```python
from build123d import *

# Parameters (mm, degrees)
SKETCH2_W           = 35.417007692
SKETCH2_H           = 35.417007691
SKETCH2_R           = 1.625
BOSS_EXTRUDE1_DEPTH = 4.975
SKETCH3_R           = 2.5
SKETCH3_R_2         = 1.625
BOSS_EXTRUDE2_DEPTH = 5.4
FILLET1_R           = 2.4
FILLET2_R           = 1


with BuildPart() as part:
    # Sketch2 → Boss-Extrude1 (new body)
    with BuildSketch(Plane.YZ):
        with Locations((28.194, 151.93658674)):
            Rectangle(SKETCH2_W, SKETCH2_H)
        with Locations(Location((16.194, 163.93658674, 0), (0, 0, 270))):
            Circle(SKETCH2_R, mode=Mode.SUBTRACT)
        with Locations(Location((40.194, 163.93658674, 0), (0, 0, 270))):
            Circle(SKETCH2_R, mode=Mode.SUBTRACT)
        with Locations(Location((40.194, 139.93658674, 0), (0, 0, 270))):
            Circle(SKETCH2_R, mode=Mode.SUBTRACT)
        with Locations(Location((16.194, 139.93658674, 0), (0, 0, 270))):
            Circle(SKETCH2_R, mode=Mode.SUBTRACT)
    extrude(amount=BOSS_EXTRUDE1_DEPTH)

    # Sketch3 → Boss-Extrude2 (add)
    # profile 1 of 4: a face of its own
    with BuildSketch(Plane.YZ.offset(4.975)):
        with Locations(Location((16.194, 163.93658674, 0), (0, 0, 90))):
            Circle(SKETCH3_R)
        with Locations(Location((16.194, 163.93658674, 0), (0, 0, 270))):
            Circle(SKETCH3_R_2, mode=Mode.SUBTRACT)
    # profile 2 of 4: a face of its own
    with BuildSketch(Plane.YZ.offset(4.975)):
        with Locations(Location((40.194, 163.93658674, 0), (0, 0, 90))):
            Circle(SKETCH3_R)
        with Locations(Location((40.194, 163.93658674, 0), (0, 0, 270))):
            Circle(SKETCH3_R_2, mode=Mode.SUBTRACT)
    # profile 3 of 4: a face of its own
    with BuildSketch(Plane.YZ.offset(4.975)):
        with Locations(Location((40.194, 139.93658674, 0), (0, 0, 90))):
            Circle(SKETCH3_R)
        with Locations(Location((40.194, 139.93658674, 0), (0, 0, 270))):
            Circle(SKETCH3_R_2, mode=Mode.SUBTRACT)
    # profile 4 of 4: a face of its own
    with BuildSketch(Plane.YZ.offset(4.975)):
        with Locations(Location((16.194, 139.93658674, 0), (0, 0, 90))):
            Circle(SKETCH3_R)
        with Locations(Location((16.194, 139.93658674, 0), (0, 0, 270))):
            Circle(SKETCH3_R_2, mode=Mode.SUBTRACT)
    extrude(amount=BOSS_EXTRUDE2_DEPTH)

    # Fillet1
    fillet1_edges = [part.edges().sort_by_distance(p)[0] for p in [
        (2.4875, 10.485496154, 169.645090586),
        (2.4875, 45.902503846, 169.645090586),
        (2.4875, 45.902503846, 134.228082895),
        (2.4875, 10.485496154, 134.228082895),
    ]]
    fillet(fillet1_edges, radius=FILLET1_R)

    # Fillet2
    fillet2_edges = [part.edges().sort_by_distance(p)[0] for p in [
        (4.975, 16.194, 161.43658674),
        (4.975, 40.194, 161.43658674),
        (4.975, 40.194, 137.43658674),
        (4.975, 16.194, 137.43658674),
        (4.975, 28.194, 169.645090586),
        (4.975, 45.902503846, 151.93658674),
        (4.975, 10.485496154, 151.93658674),
        (4.975, 28.194, 134.228082895),
        (4.975, 11.18843988, 168.942146861),
        (4.975, 11.18843988, 134.93102662),
        (4.975, 45.19956012, 134.93102662),
        (4.975, 45.19956012, 168.942146861),
    ]]
    fillet(fillet2_edges, radius=FILLET2_R)


solid = part.part
```
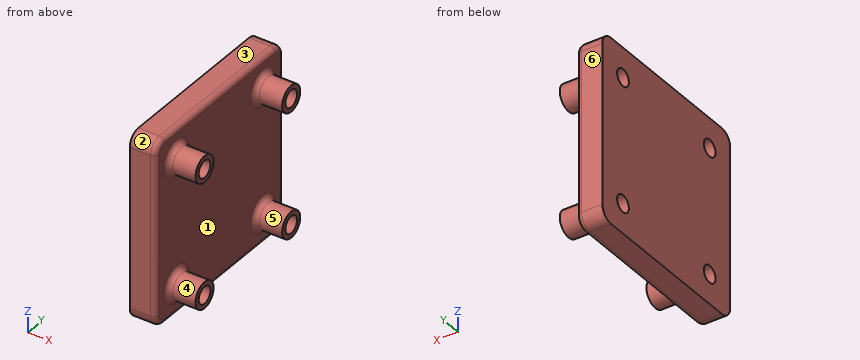
Can you work these out from the model? Positions are in its coordinate system, mm. Face numbers are marked on the shaded views. A direction names the side the tool comes from. Round coordinates to 2 decimals unless told otherwise and drop trailing zeros. Order: outer loops, then holes, each group sorted by start corner. A loop starts at its lowest first (then second) coordinate and runs counter-clockwise, first axis right, second up. Notation, with made-up numbers: (-30, 50) -> (-8, 50) arc R22 ccw to (-8, 65) -> close; hole circle Ø11 at (66, 8.5). An arc over 180 degrees is marked (long way). Return JSON: item names as keys, results as strings. Group by question number.
1. Which directions (+Z, -Z, +X, -X, +Y, -Y) give clear straight access to the entire face, cutting with the end or side of a thin tool? Please do the marked faces 5 and 6.
2. I need wall thicknesses on line 1 (Y direction, x = 7, z = 138.5); line 2 (Z direction, x = 2.5, y = 40); line 3 (X direction, y = 32.5, z = 143) (3 decimals). Which ranges of each line are inside material? Lowest first, please. Write a range as [from, to].
3. If we section it at A-A, the plane x = 7.5: Write out the boundary of the cut face in (y, z) (3 decimals).
4. We'd pull the mould along Y, two halves only. Please class the marked faces 1, 2, 3 and 4: released by +Y, released by -Y, zero draft, split by the parting line, or undercut.
5. If we section it at D-D, the plane x = 1: Count the separate pieces of the cut face and the enclosed holes in it, then the cut area to 3 significant figures.
6. If we section it at B-B, the plane y = 22.5: Write out the boundary of the cut face in (x, z) (3 decimals).
7. Will these pins go through, and if not, where does the flat tip stop? pin 1 (2.5 mm diameter, centred on y = 16.19, z = 163.94, fed in from +X); pin 2 (10 mm diameter, centred on y = 31, z = 161.5, fed in from +X) (3 decimals); pin 3 (2 mm diameter, centred on x = 9, y = 18.5, fed in from -Z).
8. If we section it at C-C, the plane z = 146.5: Write out the boundary of the cut face in (x, y) (1 decimal).
Output values:
{
 "1": {"face 5": "+X", "face 6": "+Z, -Z, +X, -X, +Y"},
 "2": {"line 1": "[14.15, 15.43], [16.95, 18.24], [38.15, 39.43], [40.95, 42.24]", "line 2": "[134.23, 138.32], [141.55, 162.32], [165.55, 169.65]", "line 3": "[0, 4.975]"},
 "3": {"outline": "circle Ø5 at (16.194, 139.937); circle Ø5 at (16.194, 163.937); circle Ø5 at (40.194, 139.937); circle Ø5 at (40.194, 163.937); hole circle Ø3.25 at (16.194, 139.937); hole circle Ø3.25 at (16.194, 163.937); hole circle Ø3.25 at (40.194, 139.937); hole circle Ø3.25 at (40.194, 163.937)"},
 "4": {"face 1": "undercut", "face 2": "released by -Y", "face 3": "zero draft", "face 4": "undercut"},
 "5": {"separate pieces": "1", "enclosed holes": "4", "area": "1,220 mm²"},
 "6": {"outline": "(0, 134.228) -> (3.975, 134.228) arc R1 ccw to (4.975, 135.228) -> (4.975, 168.645) arc R1 ccw to (3.975, 169.645) -> (0, 169.645) -> close"},
 "7": {"pin 1": "through", "pin 2": "x = 4.975", "pin 3": "z = 137.8"},
 "8": {"outline": "(0, 10.5) -> (4, 10.5) arc R1 ccw to (5, 11.5) -> (5, 44.9) arc R1 ccw to (4, 45.9) -> (0, 45.9) -> close"}
}
